from build123d import *

# Parameters (mm, degrees)
SKETCH1_R           = 21.453903958
SKETCH1_R_2         = 28.605205278
SKETCH1_R_3         = 32.180855938
SKETCH1_R_4         = 37.901896993
SKETCH1_R_5         = 42.907807917
SKETCH1_R_6         = 5.36347599
SKETCH1_R_7         = 7.721787304
BOSS_EXTRUDE1_DEPTH = 6.35


with BuildPart() as part:
    # Sketch1 → Boss-Extrude1 (new body)
    with BuildSketch(Plane(origin=(6.35, 0, 0), x_dir=(0, 0, -1), z_dir=(1, 0, 0))):
        with BuildLine():
            Line((0, 14.302602639), (0, 154.924676439))
            ThreePointArc((0, 154.924676439), (-5.001080355, 165.789579819), (-16.506943305, 169.05638987))
            Line((-16.506943305, 169.05638987), (-556.724944278, 84.790280581))
            ThreePointArc((-556.724944278, 84.790280581), (-614.910173951, 47.589388665), (-626.846614509, -20.432289484))
            Line((-626.846614509, -20.432289484), (-554.875036537, -365.59476496))
            ThreePointArc((-554.875036537, -365.59476496), (-537.95714064, -376.674692686), (-526.877212914, -359.756796789))
            Line((-526.877212914, -359.756796789), (-557.365265272, -31.595263427))
            ThreePointArc((-557.365265272, -31.595263427), (-550.174572585, -9.464586925), (-528.916762301, 0))
            Line((-528.916762301, 0), (-14.302602639, 0))
            ThreePointArc((-14.302602639, 0), (-4.189135324, 4.189135324), (0, 14.302602639))
        make_face()
        with Locations((-527.810296047, 44.736567742)):
            Circle(SKETCH1_R, mode=Mode.SUBTRACT)
        with Locations((-442.267958292, 51.579693661)):
            Circle(SKETCH1_R_2, mode=Mode.SUBTRACT)
        with Locations((-349.597092391, 58.993080074)):
            Circle(SKETCH1_R_3, mode=Mode.SUBTRACT)
        with Locations((-242.669170198, 67.546987473)):
            Circle(SKETCH1_R_4, mode=Mode.SUBTRACT)
        with Locations((-121.484191712, 77.241415858)):
            Circle(SKETCH1_R_5, mode=Mode.SUBTRACT)
        with Locations((-14.302602639, 133.35)):
            Circle(SKETCH1_R_6, mode=Mode.SUBTRACT)
        with Locations((-14.302602639, 82.55)):
            Circle(SKETCH1_R_6, mode=Mode.SUBTRACT)
        with Locations((-14.302602639, 31.75)):
            Circle(SKETCH1_R_6, mode=Mode.SUBTRACT)
        with Locations((-540.876124725, -362.675780874)):
            Circle(SKETCH1_R_7, mode=Mode.SUBTRACT)
    extrude(amount=-BOSS_EXTRUDE1_DEPTH)


solid = part.part
Geometry check sheet. Reference: the model listing, model coordinates, mm. A direction names the side the tool comes from. Round coordinates to 2 decimals unless told otherwise and drop trailing zeros. Order: outer loops, then holes, each group sorted by start corner. A loop starts at its lowest first (then second) coordinate and runs counter-clockwise, first axis right, second up. Notation, with made-up numbers: M 24,66 L 31,66 A32 cw 31,95 Z; hole C 80.5,77.25 d2. An arc over 180 degrees is marked long. Answer in a Markdown table with one row per item.
(1) Tool access check on faces 1 (the face through (3.22, -197.97, 541.91)), 2 (the face through (3.219, 53.03, 207.657)). Record the directions out of +Z, -Z, +X, -X, +Y, -Y that give a thin tool (end or side, any length) a straight path to the whole face; none if there is none.
Responses:
| item | result |
|---|---|
| face 1 | -Z, +X, -X |
| face 2 | +X, -X |
(2) Sectioned sample at C-C, the plane y = -256.5. Record the cut outline in (x, z).
Responses:
| item | result |
|---|---|
| outline | M 0,536.47 L 6.35,536.47 L 6.35,577.62 L 0,577.62 Z |
(3) Scan lines: probe 1 along Y at (x, z) = (5, 371.5); probe 2 along Y at (x, z) = (5.5, 251); probe 3 along Y at (x, z) = (2.5, 39). Record each from-to range of solid material in increasing order. Write a range as from..to.
Responses:
| item | result |
|---|---|
| probe 1 | y = 0..35.42, 82.57..113.68 |
| probe 2 | y = 0..30.57, 104.52..132.48 |
| probe 3 | y = 0..165.55 |
(4) Go/stop test with flat-tipped pins: P1, Ø18, axis at y = -362.68, z = 540.88, coming from the +X side; P2, Ø2, axis at x = 4, z = 560.5, coming from the +Y side; P3, Ø3, axis at x = 3, z = 473, coming from the -Y side; P4, Ø8.5, axis at y = 82.55, z = 14.3, coming from the +X side. Record where each tip stops, or that it passes through.
Responses:
| item | result |
|---|---|
| P1 | stops at x = 6.35 |
| P2 | stops at y = 84.31 |
| P3 | stops at y = 0 |
| P4 | passes through |
(5) Sectioned sample at A-A, the plane z = 235. Record the cut outline in (x, y), and give its area (3 significant figures).
Responses:
| item | result |
|---|---|
| outline | M 0,0 L 6.35,0 L 6.35,30.43 L 0,30.43 Z; M 0,104.66 L 6.35,104.66 L 6.35,134.97 L 0,134.97 Z |
| area | 386 mm² |
(6) Draft check along Y on faces 3 (the face through (3.2, 165.7, 4.9)), 4 (the face through (3.219, 68.659, 318.902)), 5 (the face through (3.22, 4.08, 4.3)), 6 (the face through (3.22, -365.63, 533.74)). Enter one of: released by +Y, released by -Y, zero draft, split by the parting line, or undercut.
Responses:
| item | result |
|---|---|
| face 3 | released by +Y |
| face 4 | undercut |
| face 5 | released by -Y |
| face 6 | undercut |
(7) Sectioned sample at B-B, the plane x = 2. State how many separate pieces and enclosed holes the cut face has, and give its area (3 significant figures).
Responses:
| item | result |
|---|---|
| separate pieces | 1 |
| enclosed holes | 9 |
| area | 76,500 mm² |
(8) Sectioned sample at D-D, the plane z = 572.5. Record the cut outline in (x, y).
Responses:
| item | result |
|---|---|
| outline | M 0,-281.07 L 6.35,-281.07 L 6.35,80.77 L 0,80.77 Z |
